Input: part model. Units: mm. Frame: model coordinates. A direction names the side the tool comes from. Give positions to 0.01 mm unless a question says otherwise; leave off trailing zeros. Loops run counter-clockwise (first coordinate to the right, second up) from the corner with the lowest first, then second, coordinate; pieces in that order, holes last. Notation, with made-up numbers: M 46,-12.75 L 83,-12.75 A19 cw 83,6.25 Z; hole C 5,-38 d3. An arc over 180 degrees is marked long. Use a Markdown table: item, result. Add a question column.
from build123d import *

# Parameters (mm, degrees)
SKETCH1_W           = 20
SKETCH1_H           = 23.7
BOSS_EXTRUDE1_DEPTH = 3.175
SKETCH2_W           = 7
SKETCH2_H           = 2.3
BOSS_EXTRUDE2_DEPTH = 3.175
SKETCH3_W           = 0.45
SKETCH3_H           = 23.7
CUT_EXTRUDE1_DEPTH  = 10


with BuildPart() as part:
    # Sketch1 → Boss-Extrude1 (new body)
    with BuildSketch(Plane.XY):
        with Locations((10, 11.85)):
            Rectangle(SKETCH1_W, SKETCH1_H)
    extrude(amount=BOSS_EXTRUDE1_DEPTH)

    # Sketch2 → Boss-Extrude2 (add)
    with BuildSketch(Plane.XY.offset(3.175)):
        with Locations((10.002051165, 24.85)):
            Rectangle(SKETCH2_W, SKETCH2_H)
        with Locations((10, -1.15)):
            Rectangle(SKETCH2_W, SKETCH2_H)
    extrude(amount=-BOSS_EXTRUDE2_DEPTH)

    # Sketch3 → Cut-Extrude1 (cut)
    with BuildSketch(Plane.XY.offset(3.175)):
        with Locations((0.225, 11.85)):
            Rectangle(SKETCH3_W, SKETCH3_H)
    extrude(amount=-CUT_EXTRUDE1_DEPTH, mode=Mode.SUBTRACT)


solid = part.part
1) Section query A-A, the plane z = 1.65. Return the cut outline in (x, y).
2) Contact query for flat-ended pins moving along their axis: P1, Ø1, axis at x = 15.5, z = 2.5, coming from the +Y side; P2, Ø0.7, axis at y = -1, z = 2, coming from the -X side; P3, Ø1.1, axis at y = 24.5, z = 1.5, coming from the +X side. Output: stop coordinate, or through.
3) Ray query, line 1 (Y direction, x = 16.75, z = 2.9); line 2 (X direction, y = 24.5, z = 3). Return the intervals inside material, ascending. Write a range as [from, to].
4) Section query B-B, the plane x = 15. Return the cut outline in (y, z) (3 decimals).
5) Reachability of faces 1 (the flat face through (3, 23.7, 2)), 2 (the flat face through (3, 0, 2)), 3 (the flat face through (13.5, -1, 2)), 4 (the flat face through (13.502, 25, 2)) from +Z, -Z, +X, -X, +Y, -Y: full face, straight path, thin tool, end or side. Return the list, or none.
Entries:
| question | item | result |
|---|---|---|
| 1 | outline | M 0.45,0 L 6.5,0 L 6.5,-2.3 L 13.5,-2.3 L 13.5,0 L 20,0 L 20,23.7 L 13.5,23.7 L 13.5,26 L 6.5,26 L 6.5,23.7 L 0.45,23.7 Z |
| 2 | P1 | stops at y = 23.7 |
| 2 | P2 | stops at x = 6.5 |
| 2 | P3 | stops at x = 13.5 |
| 3 | line 1 | y = [0, 23.7] |
| 3 | line 2 | x = [6.5, 13.5] |
| 4 | outline | M 0,0 L 23.7,0 L 23.7,3.175 L 0,3.175 Z |
| 5 | face 1 | +Z, -Z, -X, +Y |
| 5 | face 2 | +Z, -Z, -X, -Y |
| 5 | face 3 | +Z, -Z, +X, -Y |
| 5 | face 4 | +Z, -Z, +X, +Y |
